Could you check a few things on this drawing? It's one solid part, dimensions in mm from its lowest x, y, z. Round coordinates to 2 decimals unless told otherwise and drop trailing zeros. Write each loop counter-clockwise with the first axis right and the second up, starting at its lowest first coordinate (ties: lowest second). Pieces come first, ordered by that corner, then holes. Notation, with made-up numbers: (-6, -24) -> (30, -24) arc R12 cw to (30, -5) -> close; hole circle Ø6 at (21.25, 4.5). An arc over 180 degrees is marked (long way). Answer in a Markdown table with one row per item.
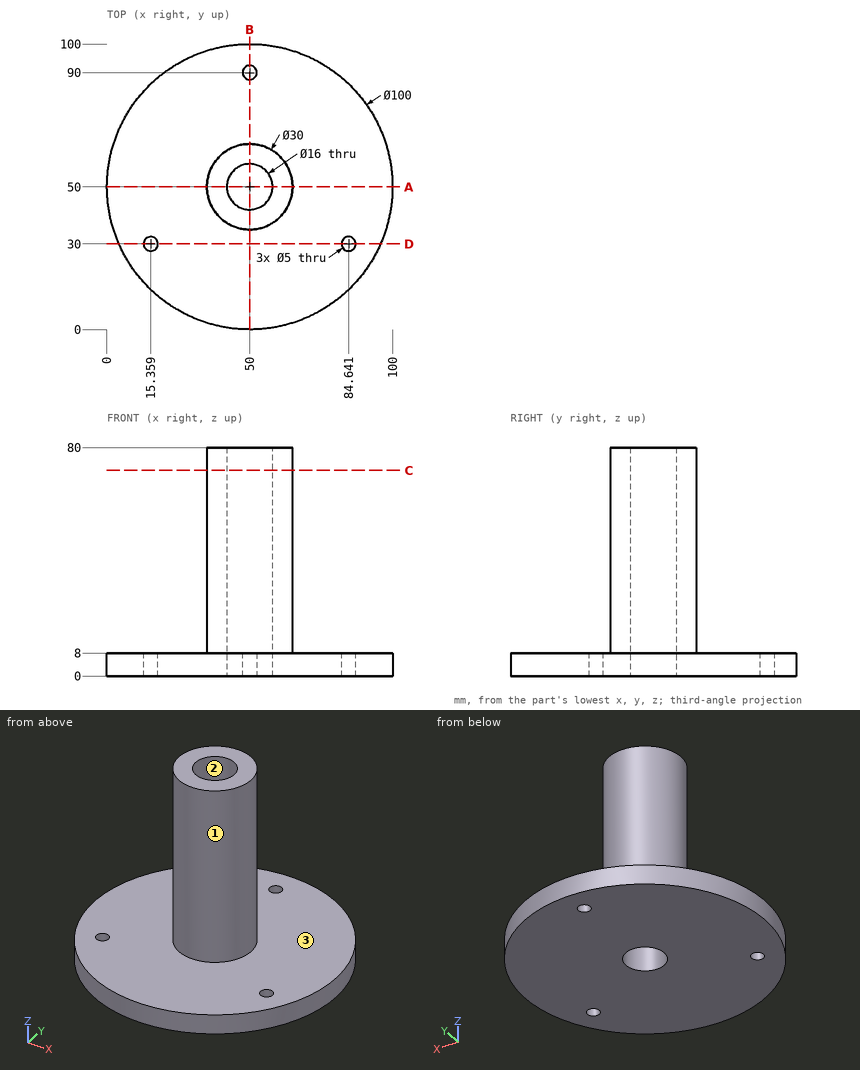
1) For pin 1 (5 mm diameter, centred on y = 53.5, z = 28.5, fed in from -X); pin 2 (2 mm diameter, centred on x = 41.5, z = 66.5, fed in from +Y); pin 3 (8 mm diameter, centred on x = 59, y = 15, fed in from +Z), each with a flat end and sliding along its axis, tell me the tip position at first contact or that it passes through.
Findings:
| item | result |
|---|---|
| pin 1 | stops at x = 35.03 |
| pin 2 | stops at y = 62.99 |
| pin 3 | stops at z = 8 |
2) Thinking about a two-plate mould opening in X: for the marked faces 1, 2 and 3, which applies, +X half, -X half, draft (parallel to the pull), parting line (faces both ways), or undercut?
Findings:
| item | result |
|---|---|
| face 1 | parting line |
| face 2 | undercut |
| face 3 | draft |
3) Imagine slicing it at C-C, the plane z = 72. Please give me the cut outline in (x, y), plus the area to 3 significant figures.
Findings:
| item | result |
|---|---|
| outline | circle Ø30 at (50, 50); hole circle Ø16 at (50, 50) |
| area | 506 mm^2 |
4) Imagine slicing it at A-A, the plane y = 50. Please give me the cut outline in (x, z), plus the area to 3 significant figures.
Findings:
| item | result |
|---|---|
| outline | (0, 0) -> (42, 0) -> (42, 80) -> (35, 80) -> (35, 8) -> (0, 8) -> close; (58, 0) -> (100, 0) -> (100, 8) -> (65, 8) -> (65, 80) -> (58, 80) -> close |
| area | 1,680 mm^2 |
5) Imagine slicing it at B-B, the plane x = 50. Please give me the cut outline in (y, z), plus the area to 3 significant figures.
Findings:
| item | result |
|---|---|
| outline | (0, 0) -> (42, 0) -> (42, 80) -> (35, 80) -> (35, 8) -> (0, 8) -> close; (58, 0) -> (87.5, 0) -> (87.5, 8) -> (65, 8) -> (65, 80) -> (58, 80) -> close; (92.5, 0) -> (100, 0) -> (100, 8) -> (92.5, 8) -> close |
| area | 1,640 mm^2 |
6) Imagine slicing it at D-D, the plane y = 30. Please give me the cut outline in (x, z).
Findings:
| item | result |
|---|---|
| outline | (4.17, 0) -> (12.86, 0) -> (12.86, 8) -> (4.17, 8) -> close; (17.86, 0) -> (82.14, 0) -> (82.14, 8) -> (17.86, 8) -> close; (87.14, 0) -> (95.83, 0) -> (95.83, 8) -> (87.14, 8) -> close |
7) Please list where these lines run through material, in increasing order: line 1 (Y direction, x = 50, z = 34); line 2 (Z direction, x = 78.5, y = 90.5); line 3 (X direction, y = 90, z = 2.25).
Findings:
| item | result |
|---|---|
| line 1 | y = 35 to 42, 58 to 65 |
| line 2 | z = 0 to 8 |
| line 3 | x = 20 to 47.5, 52.5 to 80 |
